Can you work these out from the drawing? Everything is in mm from the part's minimum corner. Round coordinates to 2 decimals unless told otherwise and drop trailing zeros. Loops run counter-clockwise (first coordinate to the right, second up) from the corner with the lowest first, then second, coordinate; pieces in that order, holes last. Notation, with made-up numbers: M 47,48.25 L 102,48.25 A21 ccw 102,85.25 Z; hole C 2,48.25 d3. An arc over 180 degrees is marked long. Return JSON: item names as keys, results as strings. Group by question number.
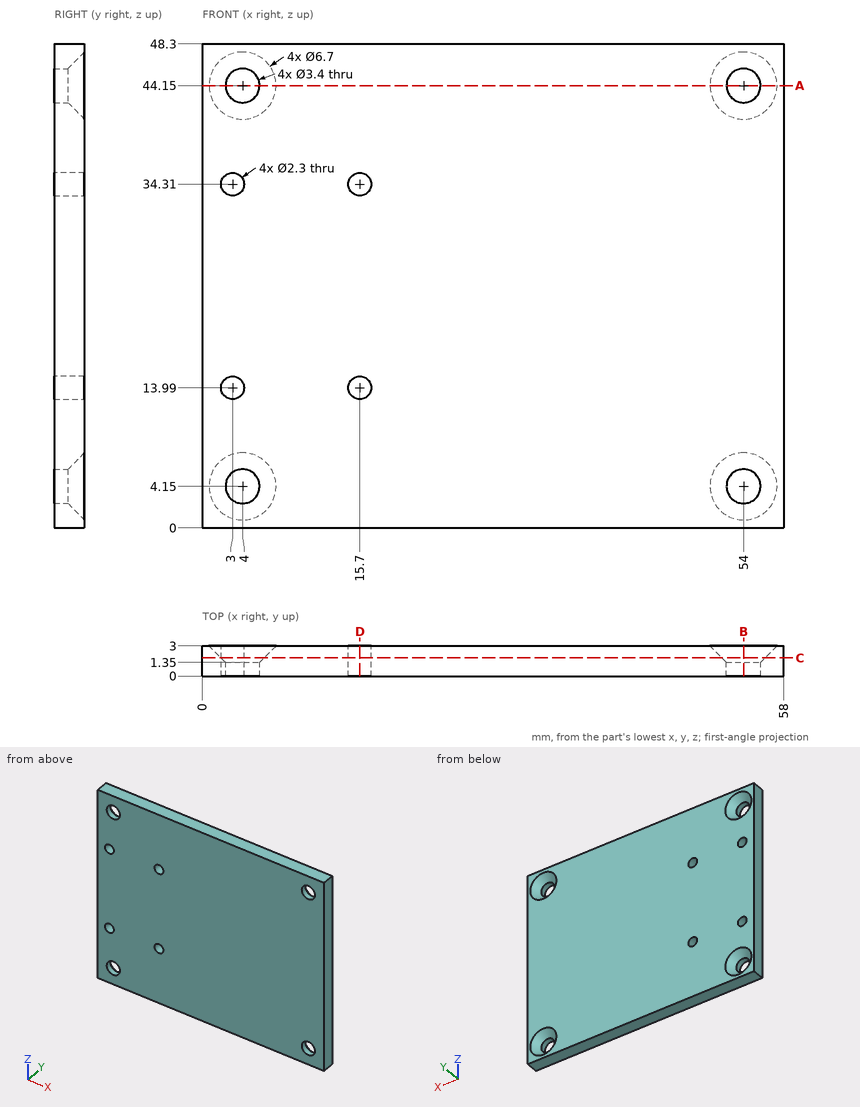
1. If we section it at B-B, the plane x = 54: Please give me the cut outline in (y, z).
2. If we section it at A-A, the plane z = 44.15: Please give me the cut outline in (x, y).
3. If we section it at C-C, the plane y = 1.8: Give the number of separate pieces and of enclosed holes in the cut face, then the cut area to 3 significant figures.
4. If we section it at D-D, the plane x = 15.7: Please give me the cut outline in (y, z).
5. I need wall thicknesses on probe 1 along X at (y, z) = (2.2, 34.31); probe 2 along Z at (x, y) = (54, 0.45); probe 3 along X at (y, z) = (0.45, 44.15). Which ranges of each line are inside material? Lowest first, please.
6. I'm going to push flat-ended pins straight in: pin 1 Ø1.5 at (x, z) = (8, 23) entering from -Y; pin 2 Ø4 at (x, z) = (54, 4.15) entering from +Y. Where does each tip first touch, or does it pass through?
Geometry results:
{
 "1": {"outline": "M 0,0 L 3,0 L 3,0.8 L 1.35,2.45 L 0,2.45 Z; M 0,5.85 L 1.35,5.85 L 3,7.5 L 3,40.8 L 1.35,42.45 L 0,42.45 Z; M 0,45.85 L 1.35,45.85 L 3,47.5 L 3,48.3 L 0,48.3 Z"},
 "2": {"outline": "M 0,0 L 2.3,0 L 2.3,1.35 L 0.65,3 L 0,3 Z; M 5.7,0 L 52.3,0 L 52.3,1.35 L 50.65,3 L 7.35,3 L 5.7,1.35 Z; M 55.7,0 L 58,0 L 58,3 L 57.35,3 L 55.7,1.35 Z"},
 "3": {"separate pieces": "1", "enclosed holes": "8", "area": "2,730 mm^2"},
 "4": {"outline": "M 0,0 L 3,0 L 3,12.84 L 0,12.84 Z; M 0,15.14 L 3,15.14 L 3,33.16 L 0,33.16 Z; M 0,35.46 L 3,35.46 L 3,48.3 L 0,48.3 Z"},
 "5": {"probe 1": "0 to 1.85, 4.15 to 14.55, 16.85 to 58", "probe 2": "0 to 2.45, 5.85 to 42.45, 45.85 to 48.3", "probe 3": "0 to 2.3, 5.7 to 52.3, 55.7 to 58"},
 "6": {"pin 1": "y = 0", "pin 2": "y = 1.65"}
}
